Part model, mm, in its own coordinate system. A direction names the side the tool comes from. Coordinates: 2 decimals unless noted, no trailing zeros. Order: outer loops, then holes, each group sorted by start corner. A loop starts at its lowest first (then second) coordinate and runs counter-clockwise, first axis right, second up. Notation, with made-up numbers: (-32, -10) - (1, -10) arc R20 cw to (1, 0) - close; hole circle Ø6 at (41, 17). An arc over 180 degrees is marked (long way). Use a Markdown table: item, result. Add a question column.
1) Saw through at C-C on z = 55. List the corners of the cut face in (x, y).
2) Saw through at A-A on z = -59.5. Count the separate pieces of the cut face and the enclosed holes in it, then the cut area to 3 significant figures.
3) Drop flat-ended pins along their axis: P1, Ø2, axis at x = 517.5, z = -83.5, coming from the -Y side; P2, Ø4, axis at x = 400, z = -11, coming from the +Y side; P3, Ø1.7, axis at y = 10, z = -12.5, coming from the -X side. Give the stop position or say it passes through.
4) Saw through at B-B on x = 469. List the corners of the cut face in (y, z), then the cut area to 3 significant figures.
5) Two-plate mould, pull along Z, no slides. Class faces 1 (the face through (639.849, -8.786, -14.393)), 2 (the face through (523, 3, -111.998)), 3 (the face through (40.211, 1, 1)), 4 (the face through (519.849, -8.786, -14.393)): +Z half, -Z half, draft (parallel to the pull), parting line (faces both ways), or undercut.
6) Wall check: L1, parallel to X at y = -7.5, z = -15; L2, parallel to X at y = 10, z = -24; L3, parallel to Y at x = 280, z = -27. Give the ranges that are in metal, low to high. Write a range as [from, to].
7) Tool access for faces 5 (the face through (276, 0, -21.998)), 6 (the face through (633, -6, -21.998)), 7 (the face through (414.518, 4.549, 67.162)): list every direction of +Z, -Z, +X, -X, +Y, -Y with a clear straight run to the whole face (end or side of a thin tool).
```python
from build123d import *

# Parameters (mm, degrees)
BOSS_EXTRUDE1_DEPTH   = 25
BOSS_EXTRUDE1_2_DEPTH = 25
BOSS_EXTRUDE1_3_DEPTH = 25
BOSS_EXTRUDE1_4_DEPTH = 25
BOSS_EXTRUDE1_5_DEPTH = 25
SKETCH3_R             = 6
CUT_EXTRUDE1_DEPTH    = 150
SKETCH11_R            = 10
SKETCH11_R_2          = 6
CUT_EXTRUDE2_DEPTH    = 150
SKETCH12_W            = 25
SKETCH12_H            = 73
BOSS_EXTRUDE2_DEPTH   = 1200
SKETCH13_R            = 25
BOSS_EXTRUDE3_DEPTH   = 200
SCALE1_SCALE          = 0.6


with BuildPart() as part:
    # Sketch1 → Boss-Extrude1 (new body)
    with BuildSketch(Plane.XY):
        with BuildLine():
            Line((4, 18), (-4, 18))
            Line((-4, 18), (-4, 14.456832295))
            ThreePointArc((-4, 14.456832295), (0, -15), (4, 14.456832295))
            Line((4, 14.456832295), (4, 18))
        make_face()
    extrude(amount=-BOSS_EXTRUDE1_DEPTH)

    # Sketch2 → Revolve1 (revolve)
    with BuildSketch(Plane(origin=(0, 0, 0), x_dir=(0, 0, -1), z_dir=(1, 0, 0)), mode=Mode.PRIVATE) as revolve1_sk:
        Polygon((25, -0.271583853), (175, -0.271583853), (175, 9.728416147), (25, 49.728416147), align=None)
    revolve(revolve1_sk.sketch.rotate(Axis((0, -0.271583853, -25), (0, 0, -1)), 180), axis=Axis((0, -0.271583853, -25), (0, 0, -1)))

    # Sketch3 → Cut-Extrude1 (cut)
    with BuildSketch(Plane(origin=(0, 0, -175), x_dir=(-1, 0, 0), z_dir=(0, 0, -1))):
        with Locations(Location((0, 0, 0), (0, 0, 90))):
            Circle(SKETCH3_R)
    extrude(amount=-CUT_EXTRUDE1_DEPTH, mode=Mode.SUBTRACT)



with BuildPart() as body_2:
    # Sketch1 → Boss-Extrude1 2 (new body)
    with BuildSketch(Plane.XY):
        with BuildLine():
            Line((204, 18), (196, 18))
            Line((196, 18), (196, 14.456832295))
            ThreePointArc((196, 14.456832295), (200, -15), (204, 14.456832295))
            Line((204, 14.456832295), (204, 18))
        make_face()
    extrude(amount=-BOSS_EXTRUDE1_2_DEPTH)

    # Sketch7 → Revolve2 (revolve)
    with BuildSketch(Plane(origin=(200, 0, 0), x_dir=(0, 0, -1), z_dir=(1, 0, 0)), mode=Mode.PRIVATE) as revolve2_sk:
        Polygon((25, -0.271583853), (175, -0.271583853), (175, 9.728416147), (25, 49.728416147), align=None)
    revolve(revolve2_sk.sketch.rotate(Axis((200, -0.271583853, -25), (0, 0, -1)), 180), axis=Axis((200, -0.271583853, -25), (0, 0, -1)))


with BuildPart() as body_3:
    # Sketch1 → Boss-Extrude1 3 (new body)
    with BuildSketch(Plane.XY):
        with BuildLine():
            Line((404, 18), (396, 18))
            Line((396, 18), (396, 14.456832295))
            ThreePointArc((396, 14.456832295), (400, -15), (404, 14.456832295))
            Line((404, 14.456832295), (404, 18))
        make_face()
    extrude(amount=-BOSS_EXTRUDE1_3_DEPTH)

    # Sketch8 → Revolve3 (revolve)
    with BuildSketch(Plane(origin=(400, 0, 0), x_dir=(0, 0, -1), z_dir=(1, 0, 0)), mode=Mode.PRIVATE) as revolve3_sk:
        Polygon((25, -0.271583853), (175, -0.271583853), (175, 9.728416147), (25, 49.728416147), align=None)
    revolve(revolve3_sk.sketch.rotate(Axis((400, -0.271583853, -25), (0, 0, -1)), 180), axis=Axis((400, -0.271583853, -25), (0, 0, -1)))


with BuildPart() as body_4:
    # Sketch1 → Boss-Extrude1 4 (new body)
    with BuildSketch(Plane.XY):
        with BuildLine():
            Line((604, 18), (596, 18))
            Line((596, 18), (596, 14.456832295))
            ThreePointArc((596, 14.456832295), (600, -15), (604, 14.456832295))
            Line((604, 14.456832295), (604, 18))
        make_face()
    extrude(amount=-BOSS_EXTRUDE1_4_DEPTH)

    # Sketch9 → Revolve4 (revolve)
    with BuildSketch(Plane(origin=(600, 0, 0), x_dir=(0, 0, -1), z_dir=(1, 0, 0)), mode=Mode.PRIVATE) as revolve4_sk:
        Polygon((25, -0.271583853), (175, -0.271583853), (175, 9.728416147), (25, 49.728416147), align=None)
    revolve(revolve4_sk.sketch.rotate(Axis((600, -0.271583853, -25), (0, 0, -1)), 180), axis=Axis((600, -0.271583853, -25), (0, 0, -1)))


with BuildPart() as body_5:
    # Sketch1 → Boss-Extrude1 5 (new body)
    with BuildSketch(Plane.XY):
        with BuildLine():
            Line((804, 18), (796, 18))
            Line((796, 18), (796, 14.456832295))
            ThreePointArc((796, 14.456832295), (800, -15), (804, 14.456832295))
            Line((804, 14.456832295), (804, 18))
        make_face()
    extrude(amount=-BOSS_EXTRUDE1_5_DEPTH)

    # Sketch10 → Revolve5 (revolve)
    with BuildSketch(Plane(origin=(800, 0, 0), x_dir=(0, 0, -1), z_dir=(1, 0, 0)), mode=Mode.PRIVATE) as revolve5_sk:
        Polygon((25, -0.271583853), (175, -0.271583853), (175, 9.728416147), (25, 49.728416147), align=None)
    revolve(revolve5_sk.sketch.rotate(Axis((800, -0.271583853, -25), (0, 0, -1)), 180), axis=Axis((800, -0.271583853, -25), (0, 0, -1)))


with BuildPart() as cut_extrude2_tool:
    # Sketch11 → Cut-Extrude2 (new body)
    # profile 1 of 5: a face of its own
    with BuildSketch(Plane(origin=(0, 0, -175), x_dir=(-1, 0, 0), z_dir=(0, 0, -1))):
        with Locations(Location((-200, -0.271583853, 0), (0, 0, 90))):
            Circle(SKETCH11_R)
        with Locations(Location((-200, -0.271583853, 0), (0, 0, 90))):
            Circle(SKETCH11_R_2, mode=Mode.SUBTRACT)
    # profile 2 of 5: a face of its own
    with BuildSketch(Plane(origin=(0, 0, -175), x_dir=(-1, 0, 0), z_dir=(0, 0, -1))):
        with Locations(Location((0, 0, 0), (0, 0, 90))):
            Circle(SKETCH11_R_2)
    # profile 3 of 5: a face of its own
    with BuildSketch(Plane(origin=(0, 0, -175), x_dir=(-1, 0, 0), z_dir=(0, 0, -1))):
        with Locations(Location((-400, -0.271583853, 0), (0, 0, 90))):
            Circle(SKETCH11_R_2)
    # profile 4 of 5: a face of its own
    with BuildSketch(Plane(origin=(0, 0, -175), x_dir=(-1, 0, 0), z_dir=(0, 0, -1))):
        with Locations(Location((-600, -0.271583853, 0), (0, 0, 90))):
            Circle(SKETCH11_R_2)
    # profile 5 of 5: a face of its own
    with BuildSketch(Plane(origin=(0, 0, -175), x_dir=(-1, 0, 0), z_dir=(0, 0, -1))):
        with Locations(Location((-800, -0.271583853, 0), (0, 0, 90))):
            Circle(SKETCH11_R_2)
    extrude(amount=-CUT_EXTRUDE2_DEPTH)


with BuildPart() as body_2_1:
    add(body_2.part)

    # Cut-Extrude2: cut by cut_extrude2_tool
    add(cut_extrude2_tool.part, mode=Mode.SUBTRACT)


with BuildPart() as body_3_1:
    add(body_3.part)

    # Cut-Extrude2: cut by cut_extrude2_tool
    add(cut_extrude2_tool.part, mode=Mode.SUBTRACT)


with BuildPart() as body_4_1:
    add(body_4.part)

    # Cut-Extrude2: cut by cut_extrude2_tool
    add(cut_extrude2_tool.part, mode=Mode.SUBTRACT)


with BuildPart() as body_5_1:
    add(body_5.part)

    # Cut-Extrude2: cut by cut_extrude2_tool
    add(cut_extrude2_tool.part, mode=Mode.SUBTRACT)


with BuildPart() as part_1:
    add(part.part)

    add(body_2_1.part)  # Boss-Extrude2 merges body 2

    add(body_3_1.part)  # Boss-Extrude2 merges body 3

    add(body_4_1.part)  # Boss-Extrude2 merges body 4

    add(body_5_1.part)  # Boss-Extrude2 merges body 5
    # Sketch12 → Boss-Extrude2 (add)
    with BuildSketch(Plane(origin=(1000, 0, 0), x_dir=(0, 0, -1), z_dir=(1, 0, 0))):
        with Locations((-12.5, 1.5)):
            Rectangle(SKETCH12_W, SKETCH12_H)
    extrude(amount=-BOSS_EXTRUDE2_DEPTH)

    # Sketch13 → Boss-Extrude3 (add)
    with BuildSketch(Plane.XY.offset(25)):
        with Locations((400, -0.271583853)):
            Circle(SKETCH13_R)
    extrude(amount=BOSS_EXTRUDE3_DEPTH)


with BuildPart() as part_2:
    # Scale1: scaled about (400.526633952, 0.517126038, -17.495206872)
    add(part_1.part.scale(SCALE1_SCALE).moved(Location((160.210653581, 0.206850415, -6.998082749))))


solid = part_2.part
```
Results are:
| question | item | result |
|---|---|---|
| 1 | outline | circle Ø30 at (400.21, 0.04) |
| 2 | separate pieces | 6 |
| 2 | enclosed holes | 5 |
| 2 | area | 6,050 mm2 |
| 3 | P1 | y = -13.61 |
| 3 | P2 | y = 11.01 |
| 3 | P3 | x = 157.81 |
| 4 | outline | (-20.79, -7) - (23.01, -7) - (23.01, 8) - (-20.79, 8) - close |
| 4 | area | 657 mm2 |
| 5 | face 1 | undercut |
| 5 | face 2 | -Z half |
| 5 | face 3 | draft |
| 5 | face 4 | undercut |
| 6 | L1 | [155.56, 164.86], [275.56, 284.86], [395.56, 404.86], [515.56, 524.86], [635.56, 644.86] |
| 6 | L2 | [132.48, 187.94], [252.48, 307.94], [372.48, 427.94], [492.48, 547.94], [612.48, 667.94] |
| 6 | L3 | [-28.62, -5.95], [-3.55, 3.64], [6.04, 28.71] |
| 7 | face 5 | -Z |
| 7 | face 6 | none |
| 7 | face 7 | +Z |
